The drawing under review shows one solid part. Ordinate dimensions are in mm from its lowest x, y, z. Give positions to 0.01 mm unless a question says otherwise; leave off trailing zeros. Order: outer loops, then holes, each group sorted by start corner. A loop starts at its lowest first (then second) coordinate and runs counter-clockwise, first axis right, second up. Notation, with made-up numbers: (-25.5, 27.5) -> (24.5, 27.5) arc R16 cw to (24.5, 44.5) -> close; hole circle Ø7 at (71, 78.5). An arc over 180 degrees is marked (long way). One line per item, written item: value. Start each with the question number.
1) Wall thickness on line 1 along X through (y, z) = (0.25, 11.8); line 2 along X through (y, z) = (0.3, 9.5); line 3 along Z through (x, y) = (15, 0.1): over which ranges is each line inside the solid? List them lowest first. Write a range as from..to.
2) Consider section C-C (x = 11.8). State the section outline as (y, z) points.
3) Consider section A-A (z = 11.8). State the section outline as (x, y) points.
4) Consider section D-D (x = 21.25). State the section outline as (y, z) points.
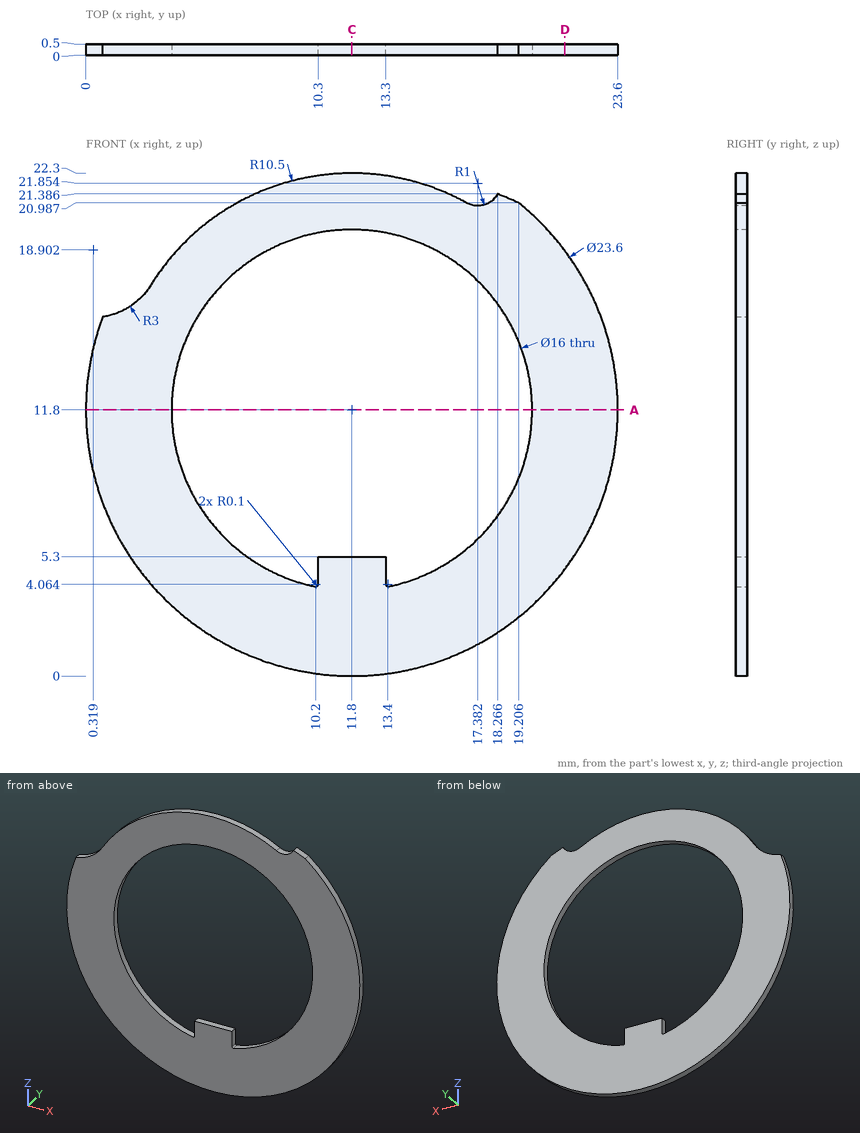
Checked values:
1. line 1: x = 0..3.8, 19.8..23.6
1. line 2: x = 0.23..4.14, 19.46..23.37
1. line 3: z = 0.44..4.47, 19.13..21.8
2. outline: (0, 0) -> (0.5, 0) -> (0.5, 5.3) -> (0, 5.3) -> close; (0, 19.8) -> (0.5, 19.8) -> (0.5, 22.3) -> (0, 22.3) -> close
3. outline: (0, 0) -> (3.8, 0) -> (3.8, 0.5) -> (0, 0.5) -> close; (19.8, 0) -> (23.6, 0) -> (23.6, 0.5) -> (19.8, 0.5) -> close
4. outline: (0, 4.73) -> (0.5, 4.73) -> (0.5, 18.87) -> (0, 18.87) -> close
